For this review, take the finished solid that the model builds, in its own axes (mm). A direction names the side the tool comes from. Coordinates: 2 decimals unless noted, no trailing zeros. Write each loop counter-clockwise with the first axis right and the second up, starting at its lowest first coordinate (ties: lowest second). Pieces come first, ordered by that corner, then holes. Notation, with made-up numbers: (6, -5.5) -> (44, -5.5) arc R15 ccw to (44, 1.5) -> close; hole circle Ø4 at (25.5, -9). An arc over 180 degrees is marked (long way). Put each result on its own line as item: value. Start each with the question number.
Item 1: Consider section D-D on x = 13. Give the boundary of the cut face in (y, z).
Item 2: For faces 4 (the flat face through (-5.6, -31.2, 3.3)), 5 (the flat face through (2, 0, -26)), 6 (the flat face through (0, -10, -25)), list the 3-axis set-ups (+Z, -Z, +X, -X, +Y, -Y) from which the entire face can be reached by the end or side of a thin tool; tool diameter is ignored.
Item 3: To check wall thickness, follow L1, parallel to Z at x = 16, y = -10.5; L2, parallel to Z at x = 0, y = -26; L3, parallel to X at y = -38, z = 0. State the ranges of each line that lie inside material, in increasing order.
Item 4: Consider section C-C on z = -17. Give the boundary of the cut face in (x, y).
Item 5: Consider section B-B on y = -35.5. Give the boundary of the cut face in (x, z), and give its area (3 significant figures).
Item 6: The part is to be moulded in two halves that separate along Z. For faces 1 (the flat face through (0, -31, 6.5)), 2 (the flat face through (27, -20, 0)), 3 (the flat face through (0, -20, 27)), say which applies: +Z half, -Z half, draft (parallel to the pull), parting line (faces both ways), or undercut.
Item 7: Consider section A-A on x = 0. Give the boundary of the cut face in (y, z), and give its area (3 significant figures).
Item 8: Insertion check: P1, Ø5, axis at x = 2.5, z = 1, coming from the -Y side; P2, Ø13, axis at x = 0, z = 0, coming from the +Y side. Each pin has a flat end and moves straight along its axis. Give the tip position at first contact, or say it passes through.
```python
from build123d import *

# Parameters (mm, degrees)
BOSS_EXTRUDE1_DEPTH = 25
SKETCH2_W           = 54
SKETCH2_H           = 28
BOSS_EXTRUDE2_DEPTH = 2
SKETCH3_W           = 54
SKETCH3_H           = 28
BOSS_EXTRUDE3_DEPTH = 2
SKETCH4_R           = 4.05
CUT_EXTRUDE2_DEPTH  = 48.349762407
SKETCH5_W           = 54
SKETCH5_H           = 54
BOSS_EXTRUDE4_DEPTH = 13.5
SKETCH6_R           = 8
CUT_EXTRUDE3_DEPTH  = 7


with BuildPart() as part:
    # Sketch1 → Boss-Extrude1 (new, symmetric)
    with BuildSketch(Plane.XY):
        with BuildLine():
            Line((25, 0), (27, 0))
            Line((27, 0), (27, -28))
            Line((27, -28), (-27, -28))
            Line((-27, -28), (-27, 0))
            Line((-27, 0), (-25, 0))
            ThreePointArc((-25, 0), (0, -25), (25, 0))
        make_face()
    extrude(amount=BOSS_EXTRUDE1_DEPTH, both=True)

    # Sketch2 → Boss-Extrude2 (add)
    with BuildSketch(Plane.XY.offset(25)):
        with Locations((0, -14)):
            Rectangle(SKETCH2_W, SKETCH2_H)
    extrude(amount=BOSS_EXTRUDE2_DEPTH)

    # Sketch3 → Boss-Extrude3 (add)
    with BuildSketch(Plane(origin=(0, 0, -25), x_dir=(-1, 0, 0), z_dir=(0, 0, -1))):
        with Locations((0, -14)):
            Rectangle(SKETCH3_W, SKETCH3_H)
    extrude(amount=BOSS_EXTRUDE3_DEPTH)

    # Sketch4 → Cut-Extrude2 (cut, through all)
    with BuildSketch(Plane.XZ.offset(28)):
        with Locations(Location((0, 0, 0), (0, 0, 270))):
            Circle(SKETCH4_R)
    extrude(amount=-CUT_EXTRUDE2_DEPTH, mode=Mode.SUBTRACT)

    # Sketch5 → Boss-Extrude4 (add)
    with BuildSketch(Plane.XZ.offset(28)):
        Rectangle(SKETCH5_W, SKETCH5_H)
        Polygon((-7.505553499, 0), (-3.75277675, -6.5), (3.75277675, -6.5), (7.505553499, 0), (3.75277675, 6.5), (-3.75277675, 6.5), align=None, mode=Mode.SUBTRACT)
    extrude(amount=BOSS_EXTRUDE4_DEPTH)

    # Sketch6 → Cut-Extrude3 (cut)
    with BuildSketch(Plane.XZ.offset(41.5)):
        with Locations(Location((0, 0, 0), (0, 0, 270))):
            Circle(SKETCH6_R)
    extrude(amount=-CUT_EXTRUDE3_DEPTH, mode=Mode.SUBTRACT)


solid = part.part
```
Return value:
1. outline: (-41.5, -27) -> (0, -27) -> (0, -25) -> (-21.35, -25) -> (-21.35, 25) -> (0, 25) -> (0, 27) -> (-41.5, 27) -> close
2. face 4: -Y
2. face 5: +Z, -Z, +X, -X, +Y
2. face 6: +Y
3. L1: -27 to -25, 25 to 27
3. L2: -27 to -4.05, 4.05 to 27
3. L3: -27 to -8, 8 to 27
4. outline: (-27, -41.5) -> (27, -41.5) -> (27, 0) -> (25, 0) arc R25 cw to (-25, 0) -> (-27, 0) -> close
5. outline: (-27, -27) -> (27, -27) -> (27, 27) -> (-27, 27) -> close; hole circle Ø16 at (0, 0)
5. area: 2,710 mm^2
6. face 1: undercut
6. face 2: draft
6. face 3: +Z half
7. outline: (-41.5, -27) -> (0, -27) -> (0, -25) -> (-25, -25) -> (-25, -4.05) -> (-28, -4.05) -> (-28, -6.5) -> (-34.5, -6.5) -> (-34.5, -8) -> (-41.5, -8) -> close; (-41.5, 8) -> (-34.5, 8) -> (-34.5, 6.5) -> (-28, 6.5) -> (-28, 4.05) -> (-25, 4.05) -> (-25, 25) -> (0, 25) -> (0, 27) -> (-41.5, 27) -> close
7. area: 770 mm^2
8. P1: y = -28
8. P2: y = -24.14
